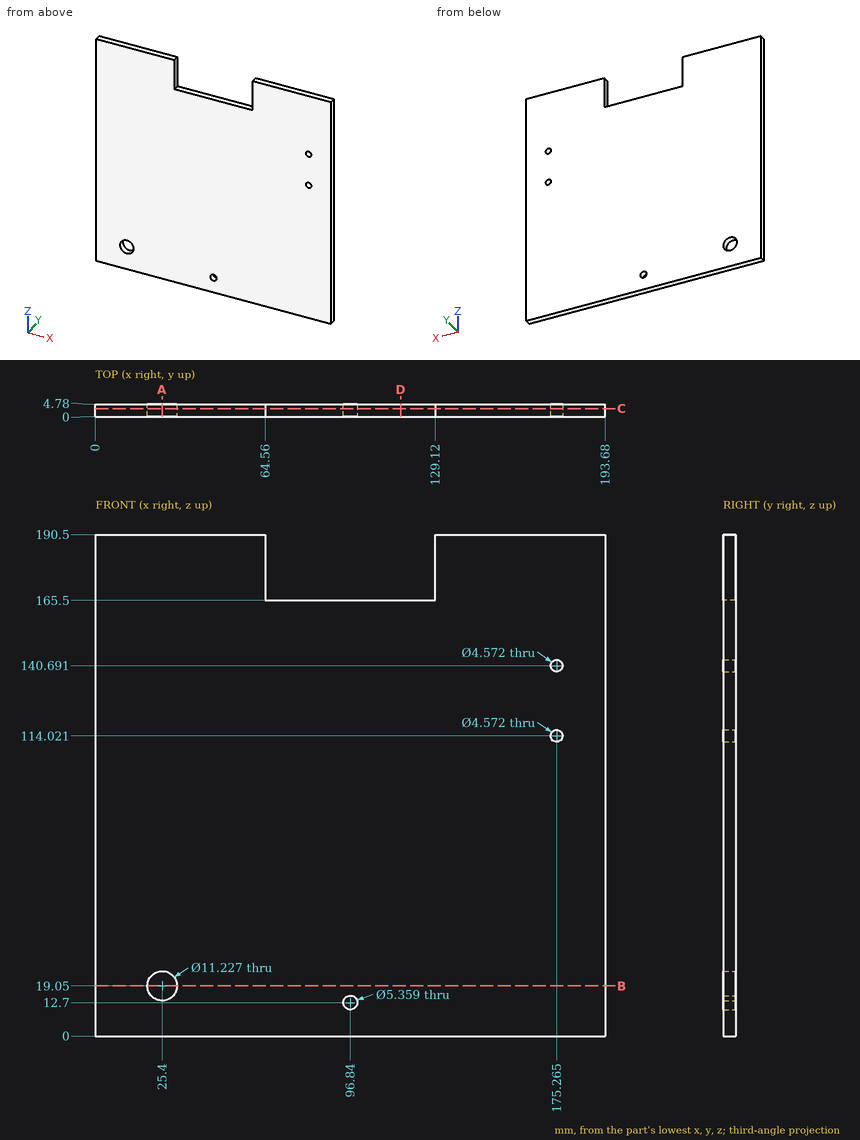
Geometry check sheet. Reference: drawing and pictorial views, mm from the part's lowest x, y, z. Give positions to 0.01 mm unless a question says otherwise; leave off trailing zeros. Order: outer loops, then holes, each group sorted by start corner. A loop starts at its lowest first (then second) coordinate and runs counter-clockwise, first axis right, second up.
1. Thickness scan on L1, parallel to X at y = 2.45, z = 177.5; L2, parallel to X at y = 4.5, z = 114; L3, parallel to Z at x = 96.84, y = 2.5. Record the ranges inside material, lowest first.
2. Section check C-C, the plane y = 3.05. Give the number of separate pieces and of enclosed holes in the cut face, and give its area (3 significant figures).
3. Gauge pin test, flat end, axial feed: pin 1 Ø10 at (x, z) = (25.4, 19.05) entering from +Y. Record the tip position at first contact, or that the pin passes through.
4. Section check B-B, the plane z = 19.05. Enter the section's corners in (x, y), and give its area (3 significant figures).
5. Section check A-A, the plane x = 25.4. Enter the section's corners in (y, z), and give its area (3 significant figures).
6. Section check D-D, the plane x = 116. Enter the section's corners in (y, z), and give its area (3 significant figures).
Values follow:
1. L1: x = 0 to 64.56, 129.12 to 193.68
1. L2: x = 0 to 172.98, 177.55 to 193.68
1. L3: z = 0 to 10.02, 15.38 to 165.5
2. separate pieces: 1
2. enclosed holes: 4
2. area: 35,100 mm2
3. pin 1: passes through
4. outline: (0, 0) - (19.79, 0) - (19.79, 4.78) - (0, 4.78) - close; (31.01, 0) - (193.68, 0) - (193.68, 4.78) - (31.01, 4.78) - close
4. area: 872 mm2
5. outline: (0, 0) - (4.78, 0) - (4.78, 13.44) - (0, 13.44) - close; (0, 24.66) - (4.78, 24.66) - (4.78, 190.5) - (0, 190.5) - close
5. area: 857 mm2
6. outline: (0, 0) - (4.78, 0) - (4.78, 165.5) - (0, 165.5) - close
6. area: 791 mm2
